Source: three-view drawing plus pictorial views. Frame: mm from the lowest corner of the part. Coordinates: 2 decimals unless noted, no trailing zeros. Order: outer loops, then holes, each group sorted by start corner. A loop starts at its lowest first (then second) coordinate and runs counter-clockwise, first axis right, second up. Notation, with made-up numbers: (53, 48) - (70, 48) arc R5 ccw to (70, 54) - close; hole circle Ø3 at (33, 69.25). An arc over 180 degrees is marked (long way). Use a Markdown table: item, result. Add a question column.
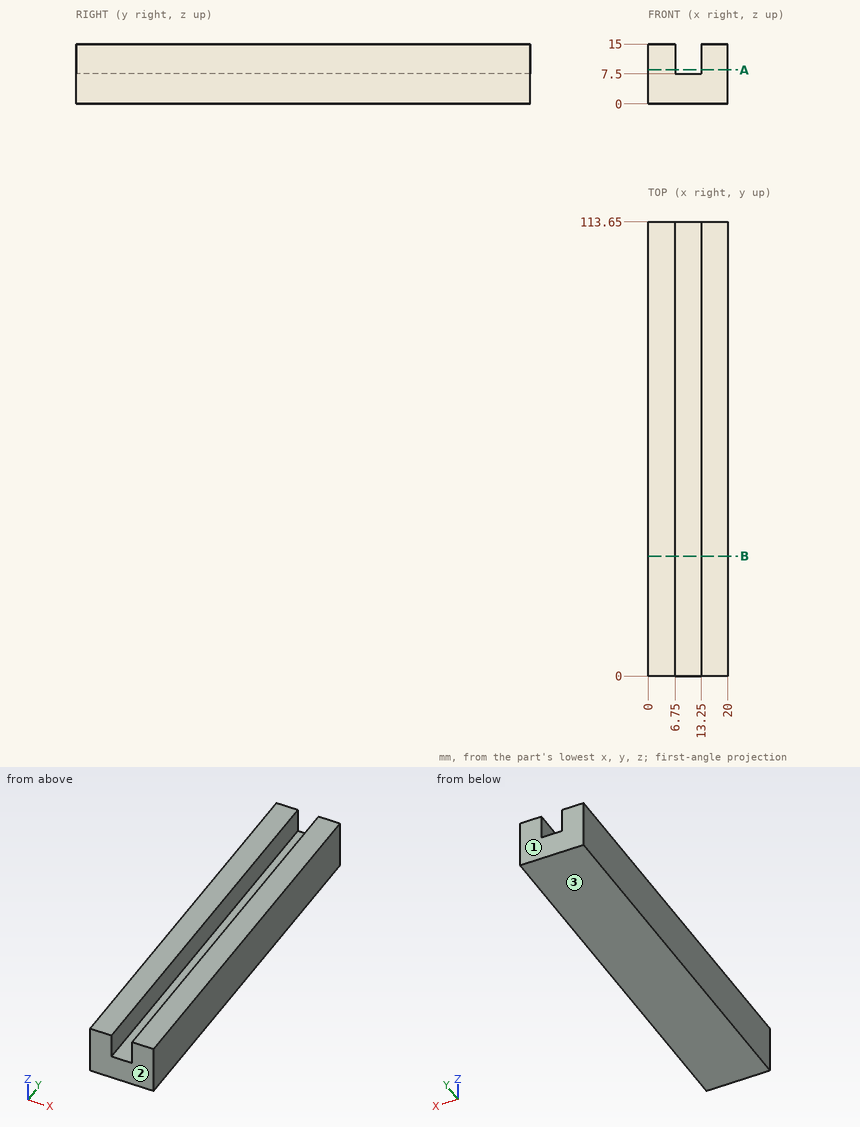
1) Pin query (flat end, axial travel): pin 1 (3 mm diameter, centred on x = 7.5, y = 34.5, fed in from -Z); pin 2 (3 mm diameter, centred on x = 10, y = 75.5, fed in from +Z). Return the tip coordinate at first contact, or that it passes through.
2) Draft query along Y for the marked faces 1, 2 and 3. Return one class per face: pulls with the +Y half, pulls with the -Y half, needs draft (parallel to the pull), parting line crosses it, or undercut.
3) Ray query, line 1 along X through (y, z) = (61, 11); line 2 along Z through (x, y) = (8.75, 6.5). Return the intervals inside material, ascending.
4) Section B-B (y = 30). Return loops of the section in (x, z).
5) Section A-A (z = 8.5). Return loops of the section in (x, y).
Values follow:
| question | item | result |
|---|---|---|
| 1 | pin 1 | stops at z = 0 |
| 1 | pin 2 | stops at z = 7.5 |
| 2 | face 1 | pulls with the +Y half |
| 2 | face 2 | pulls with the -Y half |
| 2 | face 3 | needs draft |
| 3 | line 1 | x = 0 to 6.75, 13.25 to 20 |
| 3 | line 2 | z = 0 to 7.5 |
| 4 | outline | (0, 0) - (20, 0) - (20, 15) - (13.25, 15) - (13.25, 7.5) - (6.75, 7.5) - (6.75, 15) - (0, 15) - close |
| 5 | outline | (0, 0) - (6.75, 0) - (6.75, 113.65) - (0, 113.65) - close; (13.25, 0) - (20, 0) - (20, 113.65) - (13.25, 113.65) - close |
